For this review, use the dimensioned drawing (mm, ordinates from the lowest corner) and the shaded views. Give positions to 0.01 mm unless a question says otherwise; leave off trailing zeros. Loops run counter-clockwise (first coordinate to the right, second up) from the corner with the lowest first, then second, coordinate; pieces in that order, holes last. Notation, with made-up numbers: (84.25, -14) -> (96.25, -14) arc R24 cw to (96.25, 12) -> close; hole circle Ø4 at (47, 27.25). An arc over 180 degrees is marked (long way). Use a Markdown table: item, result. Add a question column.
1. To check wall thickness, follow line 1 (Y direction, x = 12, z = 32.5) (1 decimal); line 2 (Y direction, x = 18, z = 24); line 3 (Y direction, x = 52, z = 51). State the ranges of each line that lie inside material, in increasing order.
2. Add section A-A (x = 27). State the section outline as (y, z) points (1 decimal).
3. Add section B-B (z = 58). State the section outline as (x, y) points (1 decimal).
4. Add section C-C (z = 21.5). State the section outline as (x, y) points (1 decimal), and give its area (3 significant figures).
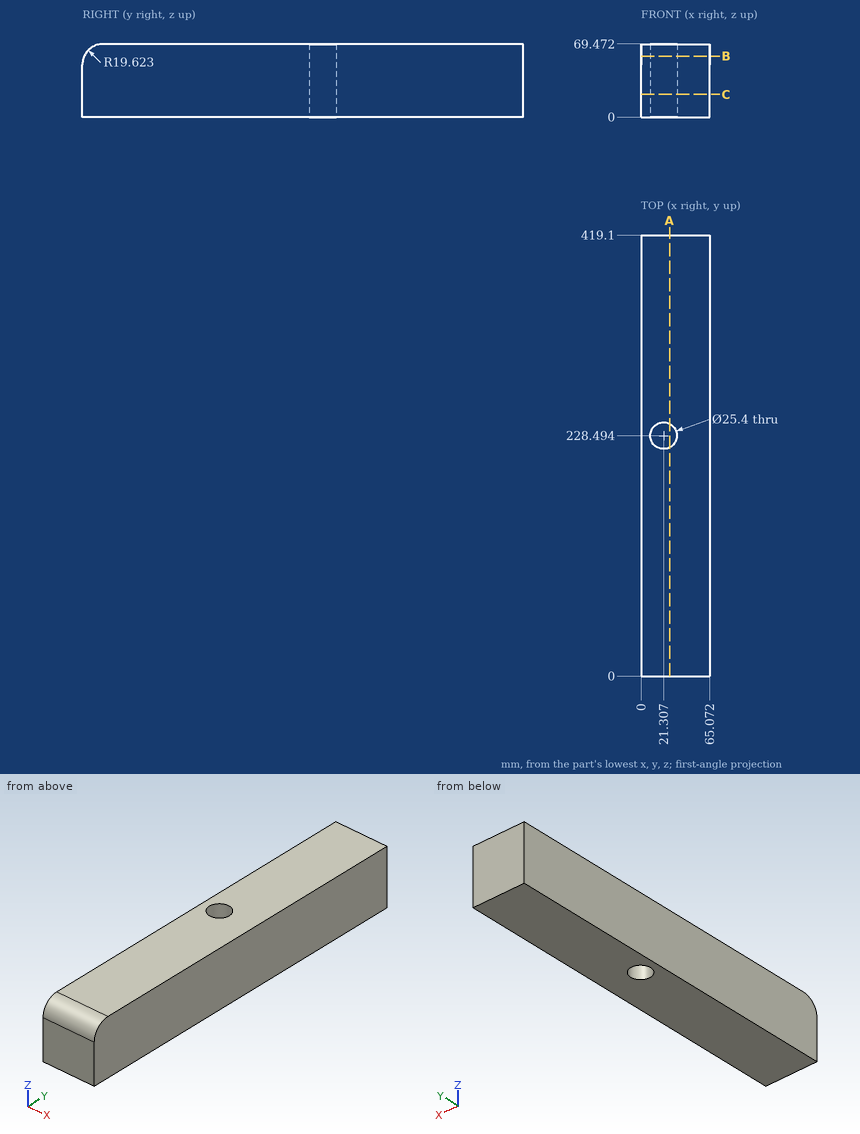
Taken from the geometry:
| question | item | result |
|---|---|---|
| 1 | line 1 | y = 0 to 219.9, 237.1 to 419.1 |
| 1 | line 2 | y = 0 to 216.23, 240.76 to 419.1 |
| 1 | line 3 | y = 0.03 to 419.1 |
| 2 | outline | (0, 0) -> (217.1, 0) -> (217.1, 69.5) -> (19.6, 69.5) arc R19.6 ccw to (0, 49.8) -> close; (239.8, 0) -> (419.1, 0) -> (419.1, 69.5) -> (239.8, 69.5) -> close |
| 3 | outline | (0, 1.8) -> (65.1, 1.8) -> (65.1, 419.1) -> (0, 419.1) -> close; hole circle Ø25.4 at (21.3, 228.5) |
| 4 | outline | (0, 0) -> (65.1, 0) -> (65.1, 419.1) -> (0, 419.1) -> close; hole circle Ø25.4 at (21.3, 228.5) |
| 4 | area | 26,800 mm^2 |
